```python
from build123d import *

# Parameters (mm, degrees)
F5_W      = 55
F5_H      = 45
F6_DEPTH  = 5
F4_W      = 53
F4_H      = 43
F7_DEPTH  = 10
F8_DEPTH  = 2
F9_R      = 2.7295
F10_DEPTH = 8
F11_D     = 2.459


with BuildPart() as f6:
    # F5 (on Top) → F6 (new body)
    with BuildSketch(Plane.XY):
        Rectangle(F5_W, F5_H)
    extrude(amount=F6_DEPTH)

    # F4 (on Top) → F7 (cut)
    with BuildSketch(Plane.XY):
        Rectangle(F4_W, F4_H)
    extrude(amount=F7_DEPTH, mode=Mode.SUBTRACT)

    # F4 (on Top) → F8 (join)
    with BuildSketch(Plane.XY):
        Rectangle(F4_W, F4_H)
    extrude(amount=F8_DEPTH)

    # F9 (on Top) → F10 (join)
    with BuildSketch(Plane.XY):
        with Locations((-16.46, 11.4)):
            Circle(F9_R)
        with Locations((14, -11.46)):
            Circle(F9_R)
        with Locations((14.0045639127, 11.4351585507)):
            Circle(F9_R)
        with Locations((-16.46, -11.3938525319)):
            Circle(F9_R)
    extrude(amount=F10_DEPTH)

    # F11 (through all)
    with Locations(Plane(origin=(0, 0, 0), x_dir=(1, 0, 0), z_dir=(0, 0, -1))):
        with Locations((-16.46, -11.4), (14, 11.46), (14.0045639127, -11.4351585507), (-16.46, 11.3938525319)):
            Hole(F11_D / 2)


solid = f6.part
```
Design review of the part built by this model. Coordinates are the model's own, in mm. A direction names the side the tool comes from. Coordinates: 2 decimals unless noted, no trailing zeros. Order: outer loops, then holes, each group sorted by start corner. A loop starts at its lowest first (then second) coordinate and runs counter-clockwise, first axis right, second up. Notation, with made-up numbers: (29, -29) - (74, -29) arc R25 ccw to (74, -9) - close; hole circle Ø2 at (-19.75, 44). An arc over 180 degrees is marked (long way). Answer in a Markdown table with one row per item.
(1) The part is to be moulded in two halves that separate along X. For faces 3 (the flat face through (15, -13, 8)), 4 (the cylindrical face through (-18.626, 9.739, 4.958)), 5 (the flat face through (27.5, 0, 2)), say which applies: released by +X, released by -X, zero draft, split by the parting line, or undercut.
Checked values:
| item | result |
|---|---|
| face 3 | zero draft |
| face 4 | undercut |
| face 5 | released by +X |
(2) Consider section A-A on z = 4. Give the number of separate pieces and of enclosed holes in the cut face, plus the area to 3 significant figures.
Checked values:
| item | result |
|---|---|
| separate pieces | 5 |
| enclosed holes | 5 |
| area | 271 mm^2 |
(3) Consider section B-B on y = -6.5. State the section outline as (x, z) points.
Checked values:
| item | result |
|---|---|
| outline | (-27.5, 0) - (27.5, 0) - (27.5, 5) - (26.5, 5) - (26.5, 2) - (-26.5, 2) - (-26.5, 5) - (-27.5, 5) - close |
(4) For faces 1 (the cylindrical face through (11.834, -13.121, 4.958)), 2 (the flat face through (0, 0, 0)), list the 3-axis set-ups (+Z, -Z, +X, -X, +Y, -Y) from which the entire face can be reached by the end or side of a thin tool; tool diameter is ignored.
Checked values:
| item | result |
|---|---|
| face 1 | +Z |
| face 2 | -Z, +X, -X, +Y, -Y |
(5) Consider section C-C on x = -11.5. State the section outline as (y, z) points, plus the area to 3 significant figures.
Checked values:
| item | result |
|---|---|
| outline | (-22.5, 0) - (22.5, 0) - (22.5, 5) - (21.5, 5) - (21.5, 2) - (-21.5, 2) - (-21.5, 5) - (-22.5, 5) - close |
| area | 96.0 mm^2 |
(6) Clearance check with a flat-ended pin moving along its axis: pin 1 (1.5 mm diameter, centred on x = -9.5, z = 6.5, fed in from +Y). State where the tip first meets the part, or that it passes through.
Checked values:
| item | result |
|---|---|
| pin 1 | through |
(7) Wall thickness on line 1 along Y through (x, z) = (-16.46, 2.5); line 2 along Y through (x, z) = (14, 2.75); line 3 along X through (y, z) = (11.4, 2.5): over which ranges is each line inside the solid? List them lowest first. Write a range as from..to.
Checked values:
| item | result |
|---|---|
| line 1 | -22.5..-21.5, -14.12..-12.62, -10.16..-8.66, 8.67..10.17, 12.63..14.13, 21.5..22.5 |
| line 2 | -22.5..-21.5, -14.19..-12.69, -10.23..-8.73, 8.71..10.21, 12.66..14.16, 21.5..22.5 |
| line 3 | -27.5..-26.5, -19.19..-17.69, -15.23..-13.73, 11.28..12.78, 15.23..16.73, 26.5..27.5 |
